Part print with two shaded views. Sizes in mm from the minimum x, y, z corner. A direction names the side the tool comes from. Round coordinates to 2 decimals unless told otherwise and drop trailing zeros. Loops run counter-clockwise (first coordinate to the right, second up) from the corner with the lowest first, then second, coordinate; pieces in that order, holes last. Notation, with made-up numbers: (58, -2) - (103, -2) arc R29 cw to (103, 28) - close; hole circle Ø10 at (34.5, 29.5). An arc over 180 degrees is marked (long way). Use a Markdown table: item, result.
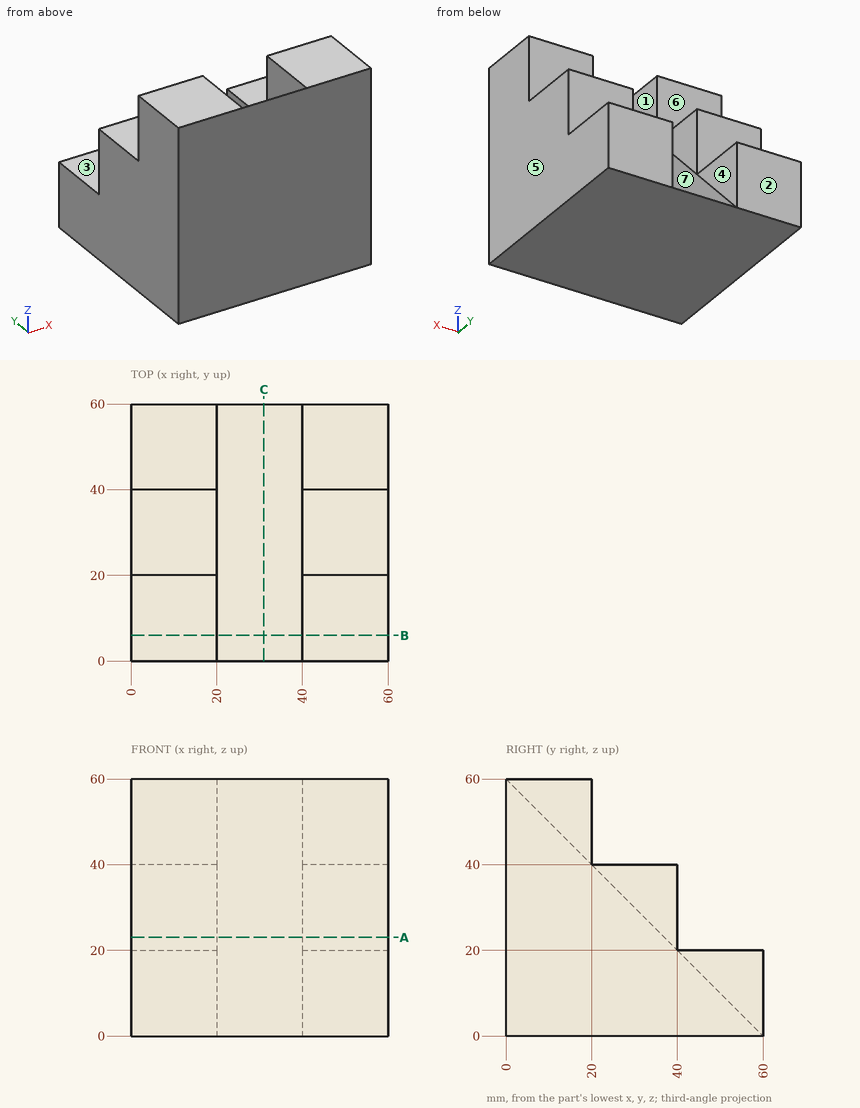
Q1. Cut at B-B, the plane y = 6. List the corners of the cut face in (x, z), plus the area to 3 significant figures.
Results found:
| item | result |
|---|---|
| outline | (0, 0) - (60, 0) - (60, 60) - (40, 60) - (40, 54) - (20, 54) - (20, 60) - (0, 60) - close |
| area | 3,480 mm2 |
Q2. Drop flat-ended pins along their axis: pin 1 (16 mm diameter, centred on x = 6.5, y = 35, fed in from +Z); pin 2 (10 mm diameter, centred on x = 9, y = 46.5, fed in from +Z); pin 3 (6 mm diameter, centred on x = 52.5, z = 29, fed in from +Y). Give the stop position or say it passes through.
Results found:
| item | result |
|---|---|
| pin 1 | stops at z = 40 |
| pin 2 | stops at z = 20 |
| pin 3 | stops at y = 40 |
Q3. Cut at A-A, the plane z = 23. List the corners of the cut face in (x, y), plus the area to 3 significant figures.
Results found:
| item | result |
|---|---|
| outline | (0, 0) - (60, 0) - (60, 40) - (40, 40) - (40, 37) - (20, 37) - (20, 40) - (0, 40) - close |
| area | 2,340 mm2 |
Q4. Probe line 1 (X direction, y = 33.5, z = 35.5); line 2 (Z direction, x = 14, y = 57.5). List the from-to ranges inside material, lowest first.
Results found:
| item | result |
|---|---|
| line 1 | x = 0 to 20, 40 to 60 |
| line 2 | z = 0 to 20 |
Q5. Cut at C-C, the plane x = 31. List the corners of the cut face in (y, z), plus the area to 3 significant figures.
Results found:
| item | result |
|---|---|
| outline | (0, 0) - (60, 0) - (0, 60) - close |
| area | 1,800 mm2 |
Q6. Pull direction X, two halves, no side cores. Call the marked faces 4, 5, 6 and 7: pulls with the +X half, pulls with the -X half, needs draft (parallel to the pull), parting line crosses it, or undercut.
Results found:
| item | result |
|---|---|
| face 4 | undercut |
| face 5 | pulls with the +X half |
| face 6 | needs draft |
| face 7 | undercut |
Q7. Which spindle directions (+Z, -Z, +X, -X, +Y, -Y) get a long thin tool onto all of the face, cutting with end or side? Do the marked faces 1, 2 and 3. Say none if no direction does.
Results found:
| item | result |
|---|---|
| face 1 | +Z, +Y |
| face 2 | +Z, -Z, +X, -X, +Y |
| face 3 | +Z, +X, -X, +Y |
